Source: three-view drawing plus pictorial views. Frame: mm from the lowest corner of the part. A direction names the side the tool comes from. Give positions to 0.01 mm unless a question says otherwise; leave off trailing zeros. Order: outer loops, then holes, each group sorted by start corner. A loop starts at its lowest first (then second) coordinate and runs counter-clockwise, first axis right, second up. Notation, with made-up numbers: (-10.5, 30) - (5.5, 30) arc R17 cw to (5.5, 58) - close; hole circle Ø1 at (46.25, 68). An arc over 180 degrees is marked (long way). Use CSV: the item, a comma, the result in double quotes.
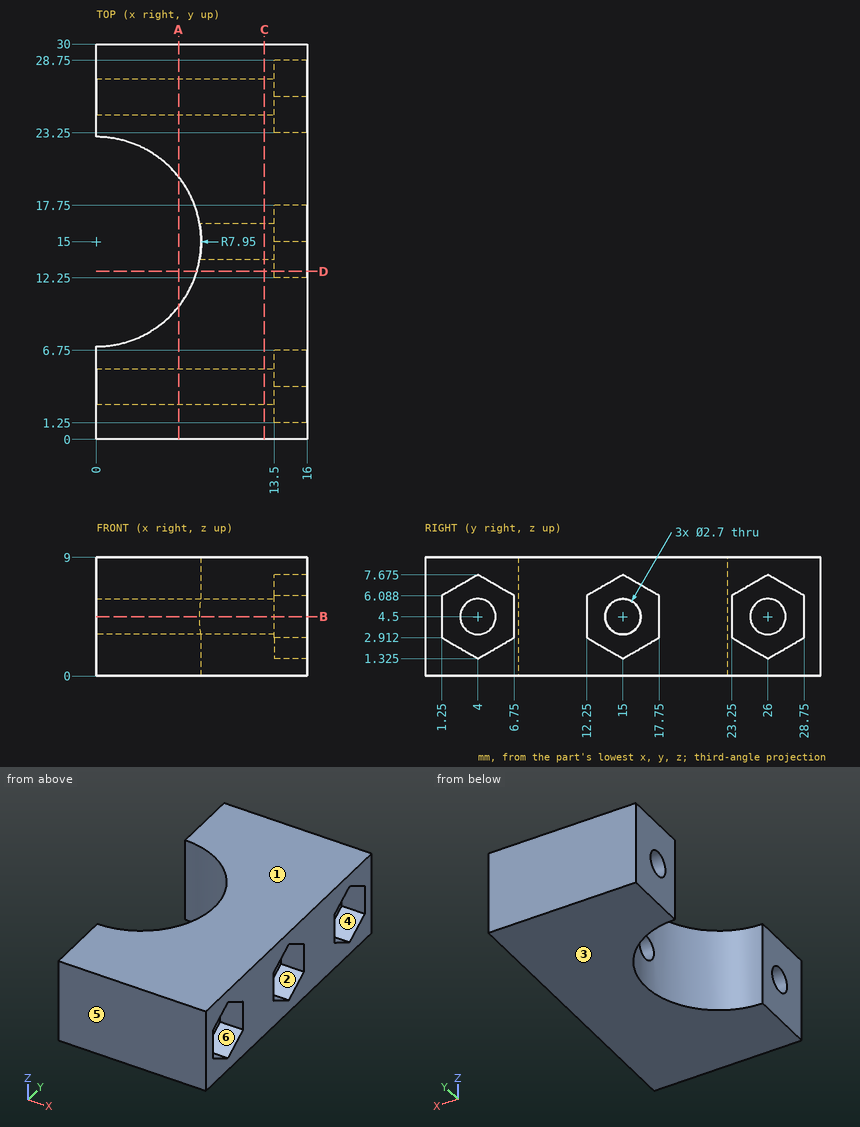
Item 1: First-contact query: pin 1 (1.6 mm diameter, centred on y = 15.5, z = 4, fed in from +X); pin 2 (3 mm diameter, centred on x = 15.5, z = 5, fed in from -Y); pin 3 (2.5 mm diameter, centred on y = 15, z = 4.5, fed in from +X). Flat tips, straight axial feed; report the tip coordinate or a pass-through.
Filled in:
pin 1,"stops at x = 13.5"
pin 2,"stops at y = 0"
pin 3,"passes through"
Item 2: Set-up query: the marked faces 1 and 2. Return all of +Z, -Z, +X, -X, +Y, -Y with unobstructed straight access to the full face (end or side cutting, diameter ignored); none if empty.
Filled in:
face 1,"+Z, +X, -X, +Y, -Y"
face 2,"+X"
Item 3: Section A-A on x = 6.25. Return the cut outline in (y, z).
Filled in:
outline,"(0, 0) - (10.09, 0) - (10.09, 9) - (0, 9) - close; (19.91, 0) - (30, 0) - (30, 9) - (19.91, 9) - close; hole circle Ø2.7 at (4, 4.5); hole circle Ø2.7 at (26, 4.5)"
Item 4: Section B-B on z = 4.5. Count the separate pieces of the cut face and the enclosed holes in it.
Filled in:
separate pieces,"4"
enclosed holes,"0"
Item 5: Mould query, pull axis Y, two halves, no side actions, for the marked faces 3, 4, 5 and 6. Classes: released by +Y, released by -Y, zero draft, split by the parting line, or undercut.
Filled in:
face 3,"zero draft"
face 4,"undercut"
face 5,"released by -Y"
face 6,"undercut"
Item 6: Material intervals for line 1 (Y direction, x = 9.5, z = 4) (1 decimal); line 2 (Y direction, x = 3.75, z = 4.5); line 3 (X direction, y = 28, z = 5), sorted ascending. Write a range as from..to.
Filled in:
line 1,"y = 0..2.7, 5.3..13.7, 16.3..24.7, 27.3..30"
line 2,"y = 0..2.65, 5.35..7.99, 22.01..24.65, 27.35..30"
line 3,"x = 0..13.5"
Item 7: Section D-D on y = 12.75. Return the cut outline in (x, z) (1 decimal).
Filled in:
outline,"(7.6, 0) - (16, 0) - (16, 2.6) - (13.5, 2.6) - (13.5, 6.4) - (16, 6.4) - (16, 9) - (7.6, 9) - close"
Item 8: Section C-C on x = 12.75. Return the cut outline in (y, z), then the cut area to 3 significant figures.
Filled in:
outline,"(0, 0) - (30, 0) - (30, 9) - (0, 9) - close; hole circle Ø2.7 at (4, 4.5); hole circle Ø2.7 at (15, 4.5); hole circle Ø2.7 at (26, 4.5)"
area,"253 mm2"
